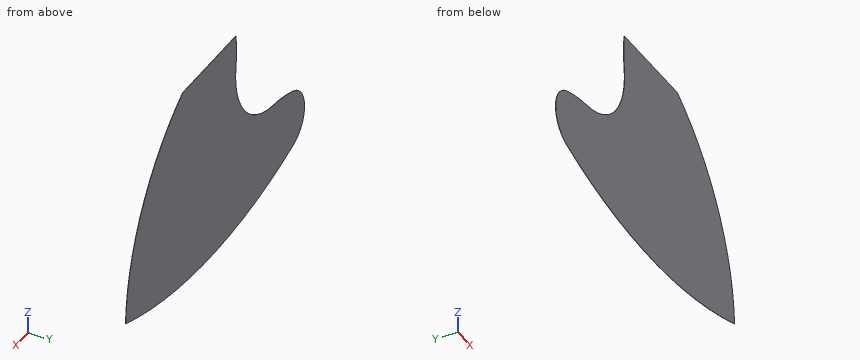
from build123d import *

# Parameters (mm, degrees)
BOSS_EXTRUDE1_DEPTH = 0.2


with BuildPart() as part:
    # Sketch1 → Boss-Extrude1 (new body)
    with BuildSketch(Plane(origin=(0, 0, 0), x_dir=(1, 0, 0), z_dir=(0, 1, 0))):
        with BuildLine():
            Line((77.011811156, 6.964256389), (142.011811156, 6.964256389))
            ThreePointArc((142.011811156, 6.964256389), (191.952101905, 59.934908511), (212.011811156, 129.917268368))
            ThreePointArc((212.011811156, 129.917268368), (109.511811156, 146.964256388), (7.011811156, 129.917268368))
            ThreePointArc((7.011811156, 129.917268368), (-6.988188844, 110.331559293), (7.011811156, 90.745850217))
            ThreePointArc((7.011811156, 90.745850217), (19.183532895, 87.425752447), (31.677095604, 85.669406772))
            ThreePointArc((31.677095604, 85.669406772), (66.484712456, 67.363163439), (77.011811156, 29.470302254))
            ThreePointArc((77.011811156, 29.470302254), (76.24065583, 18.217279321), (77.011811156, 6.964256389))
        make_face()
    extrude(amount=BOSS_EXTRUDE1_DEPTH)


solid = part.part
Geometry: final body of the model. Coordinates: model frame, mm. Coordinates: 2 decimals unless noted, no trailing zeros. Loops run counter-clockwise (first coordinate to the right, second up) from the corner with the lowest first, then second, coordinate; pieces in that order, holes last. Notation, with made-up numbers: (18.5, 89) - (77.5, 89) arc R26 ccw to (77.5, 119) - close; hole circle Ø7 at (36, -36.5). An arc over 180 degrees is marked (long way). One line per question, with ' | ' between items. Start each with the question number.
(1) Cut plane C-C on z = -54.5. Output: boundary loops of the cut face in (x, y), and give its area (3 significant figures).
(2) Cut plane A-A on y = 0.1. Output: boundary loops of the cut face in (x, z), and give its area (3 significant figures).
(3) Cut plane B-B on x = 14. Output: boundary loops of the cut face in (y, z).
(4) Ray query, L1, parallel to X at y = 0.1, z = -71; L2, parallel to X at y = 0.1, z = -82; L3, parallel to Z at x = 47, y = 0.1. Return the intervals inside material, ascending. Write a range as from..to.
Here are the results:
1) outline: (73.99, 0) - (188.71, 0) - (188.71, 0.2) - (73.99, 0.2) - close | area: 22.9 mm²
2) outline: (7.01, -129.92) arc R316.68 ccw to (212.01, -129.92) arc R154.14 ccw to (142.01, -6.96) - (77.01, -6.96) arc R82.49 ccw to (77.01, -29.47) arc R49.58 cw to (31.68, -85.67) arc R99.7 ccw to (7.01, -90.75) arc R20.7 ccw to start | area: 20,200 mm²
3) outline: (0, -132.22) - (0.2, -132.22) - (0.2, -88.64) - (0, -88.64) - close
4) L1: 63.24..197.67 | L2: 46.96..202.3 | L3: -140.73..-81.99
